Verification items for this drawing (mm, ordinates from the low corner). A direction names the side the tool comes from. Round coordinates to 2 decimals unless told otherwise and drop trailing zeros. Order: outer loops, then holes, each group sorted by start corner. A loop starts at its lowest first (then second) coordinate and runs counter-clockwise, first axis right, second up. Notation, with made-up numbers: (-39, 78) -> (9, 78) arc R27 ccw to (9, 103) -> close; hole circle Ø8 at (0.25, 30.5). An arc over 180 degrees is marked (long way). Answer in a Markdown table with one row per item.
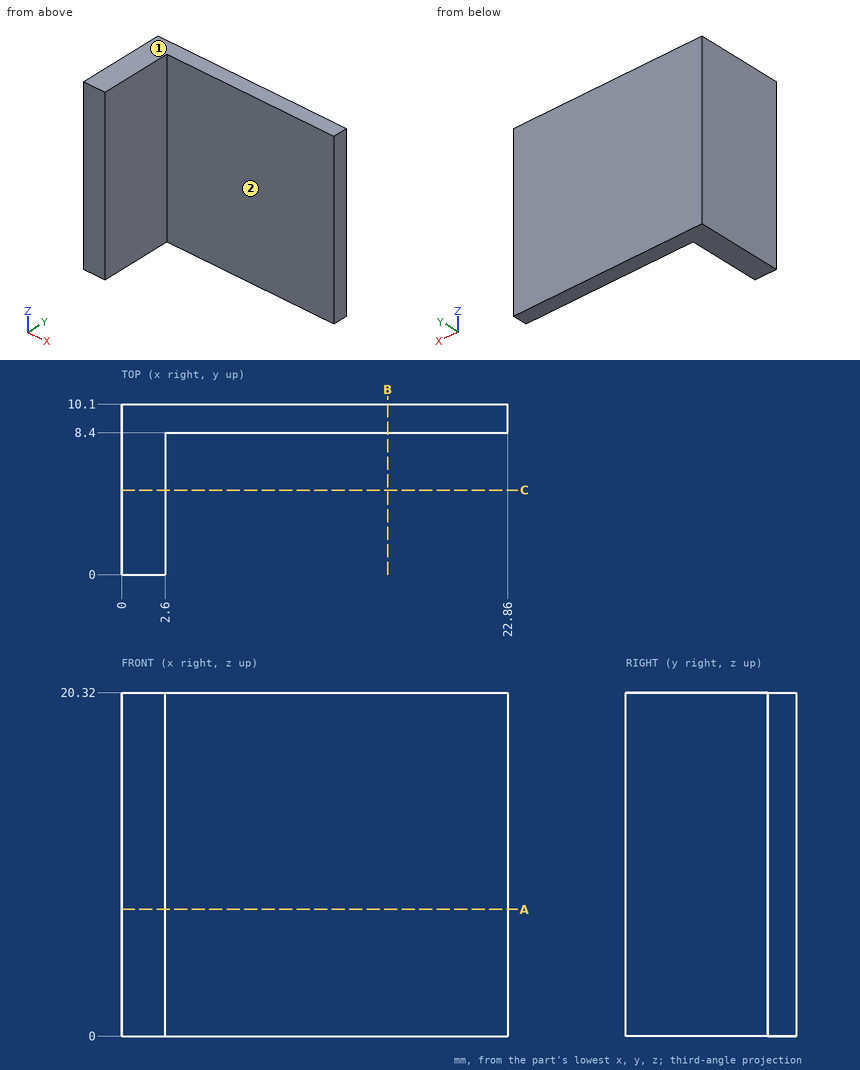
Item 1: Cross-section at C-C (y = 5). Record the boundary of the cut face in (x, z), and give its area (3 significant figures).
Result sheet:
| item | result |
|---|---|
| outline | (0, 0) -> (2.6, 0) -> (2.6, 20.32) -> (0, 20.32) -> close |
| area | 52.8 mm^2 |
Item 2: Cross-section at B-B (x = 15.75). Record the boundary of the cut face in (y, z).
Result sheet:
| item | result |
|---|---|
| outline | (8.4, 0) -> (10.1, 0) -> (10.1, 20.32) -> (8.4, 20.32) -> close |
Item 3: Set-up check for the marked faces 1 and 2: record each of +Z, -Z, +X, -X, +Y, -Y from which the full face is reachable in a straight line by a thin tool's end or side.
Result sheet:
| item | result |
|---|---|
| face 1 | +Z, +X, -X, +Y, -Y |
| face 2 | +Z, -Z, +X, -Y |
Item 4: Depth check by flat-ended pin: P1, Ø2.5, axis at y = 4, z = 6.5, coming from the +X side; P2, Ø6, axis at x = 14.5, z = 4.5, coming from the -Y side; P3, Ø1.5, axis at x = 3.5, y = 3.5, coming from the -Z side. Enter the tip coordinate at first touch or a pass-through.
Result sheet:
| item | result |
|---|---|
| P1 | stops at x = 2.6 |
| P2 | stops at y = 8.4 |
| P3 | passes through |
Item 5: Scan lines: line 1 (Y direction, x = 5.25, z = 11); line 2 (X direction, y = 7.5, z = 16.25). Record each from-to range of solid material in increasing order. Write a range as [from, to].
Result sheet:
| item | result |
|---|---|
| line 1 | y = [8.4, 10.1] |
| line 2 | x = [0, 2.6] |
Item 6: Cross-section at A-A (z = 7.5). Record the boundary of the cut face in (x, y), and give its area (3 significant figures).
Result sheet:
| item | result |
|---|---|
| outline | (0, 0) -> (2.6, 0) -> (2.6, 8.4) -> (22.86, 8.4) -> (22.86, 10.1) -> (0, 10.1) -> close |
| area | 60.7 mm^2 |
